Geometry: final body of the model. Coordinates: model frame, mm. A direction names the side the tool comes from. Round coordinates to 2 decimals unless told otherwise and drop trailing zeros. Write each loop counter-clockwise with the first axis right and the second up, starting at its lowest first coordinate (ties: lowest second). Pieces come first, ordered by that corner, then holes. Notation, with made-up numbers: (21.5, -34.75) -> (41.5, -34.75) arc R21 cw to (41.5, -19.75) -> close; hole circle Ø7 at (-11.75, 0). An arc over 180 degrees is marked (long way). Use one line per item in the form item = value. Start each with the question number.
1. Cut plane D-D, the plane y = -32. Return the cut outline in (x, z).
2. Reachability of faces 5 (the face through (5.734, -65.346, 70.392)), 6 (the face through (-5.116, -73.362, 8.112)), 7 (the face through (-8.075, -18, 2)), 8 (the face through (-6, -17, 16)) from +Z, -Z, +X, -X, +Y, -Y: full face, straight path, thin tool, end or side. Return the list, or none.
3. Draft query along Y for faces 1 (the face through (5.734, -62.007, 71.08)), 2 (the face through (-6, -77.2, 8)), 3 (the face through (-13, -46, 21)), 4 (the face through (-4, -23.65, 4)). Return one class per face: pulls with the +Y half, pulls with the -Y half, needs draft (parallel to the pull), parting line crosses it, or undercut.
4. Cut plane B-B, the plane x = -11. Return the cut outline in (y, z) (1 decimal).
5. Cut plane A-A, the plane x = -6.5. State how many separate pieces and enclosed holes the cut face has, plus the area to 3 significant figures.
6. Pin query (flat end, axial travel): pin 1 Ø10.5 at (x, y) = (-5.5, -65.5) entering from +Z; pin 2 Ø10 at (x, z) = (-3, 10.5) entering from -Y; pin 3 Ø8 at (x, y) = (-6.5, -70.7) entering from +Z. Return the tip coordinate at first contact, or that it passes through.
7. Line query: L1, parallel to Y at x = -6, z = 12; L2, parallel to Z at x = -8.5, y = -15.5; L3, parallel to X at y = -24.5, z = 3.5. Output: solid intervals per line, ascending.
```python
from build123d import *

# Parameters (mm, degrees)
F0_R      = 4.415
F0_W      = 3.025
F0_H      = 16
F0_W_2    = 7.0735459991
F1_DEPTH  = 13
F3_DEPTH  = 8.075
F4_R      = 10
F5_R      = 3
F6_DEPTH  = 25
F7_R      = 3.2
F8_DEPTH  = 11.1
F10_DEPTH = 25


# Not quite as in the source:
# - ends of sketch curves that miss each other by under 0.0002 mm in the source are joined


with BuildPart() as f1:
    # F0 (on Right) → F1 (new body)
    with BuildSketch(Plane.YZ):
        with BuildLine():
            Line((-11.2, 0), (0, 0))
            Line((0, 0), (0, 12))
            ThreePointArc((0, 12), (-1.1715728753, 14.8284271247), (-4, 16))
            Line((-4, 16), (-34.4146185314, 16))
            Line((-34.4146185314, 16), (-69.7679370642, 58.1324443715))
            Line((-69.7679370642, 58.1324443715), (-58.8383850945, 67.3034273983))
            Line((-58.8383850945, 67.3034273983), (-65.2662611913, 74.9638718294))
            Line((-65.2662611913, 74.9638718294), (-67.5643945207, 73.0355090004))
            Line((-67.5643945207, 73.0355090004), (-63.0648812529, 67.6731978986))
            Line((-63.0648812529, 67.6731978986), (-79.9178590015, 53.5318704855))
            Line((-79.9178590015, 53.5318704855), (-53.9387302293, 22.5711504387))
            ThreePointArc((-53.9387302293, 22.5711504387), (-53.3776768537, 18.309526953), (-57.0029080018, 16))
            Line((-57.0029080018, 16), (-67.1014540009, 16))
            Line((-67.1014540009, 16), (-67.1014540009, 0))
            Line((-67.1014540009, 0), (-64.0764540009, 0))
            Line((-64.0764540009, 0), (-23.65, 0))
            Line((-23.65, 0), (-23.65, 7.375))
            ThreePointArc((-23.65, 7.375), (-21.8267397129, 11.7767397129), (-17.425, 13.6))
            ThreePointArc((-17.425, 13.6), (-13.0232602871, 11.7767397129), (-11.2, 7.375))
            Line((-11.2, 7.375), (-11.2, 0))
        make_face()
        with BuildLine():
            Line((-23.65, 0), (-11.2, 0))
            Line((-11.2, 0), (-11.2, 7.375))
            ThreePointArc((-11.2, 7.375), (-13.0232602871, 11.7767397129), (-17.425, 13.6))
            ThreePointArc((-17.425, 13.6), (-21.8267397129, 11.7767397129), (-23.65, 7.375))
            Line((-23.65, 7.375), (-23.65, 0))
        make_face()
        with Locations((-17.425, 7.375)):
            Circle(F0_R, mode=Mode.SUBTRACT)
        with Locations((-68.6139540009, 8)):
            Rectangle(F0_W, F0_H)
        with Locations((-73.6632270005, 8)):
            Rectangle(F0_W_2, F0_H)
    extrude(amount=-F1_DEPTH)

    # F2 (on face) → F3 (cut)
    with BuildSketch(Plane.YZ):
        with BuildLine():
            Line((-17.425, 0), (-11.2, 0))
            Line((-11.2, 0), (-11.2, 7.3750006942))
            ThreePointArc((-11.2, 7.3750006942), (-11.2387169647, 8.068201392), (-11.3543862514, 8.7527792377))
            ThreePointArc((-11.3543862514, 8.7527792377), (-18.1182010341, 13.5612829976), (-23.65, 7.375))
            Line((-23.65, 7.375), (-23.65, 0))
            Line((-23.65, 0), (-17.425, 0))
        make_face()
        with BuildLine():
            ThreePointArc((-13.01, 7.375), (-14.3031235611, 4.2531235611), (-17.425, 2.96))
            ThreePointArc((-17.425, 2.96), (-20.5468764389, 10.4968764389), (-13.01, 7.375))
        make_face(mode=Mode.SUBTRACT)
    extrude(amount=-F3_DEPTH, mode=Mode.SUBTRACT)

    # F4
    f4_edges = [f1.edges().sort_by_distance(p)[0] for p in [
        (-6.5, -34.414619, 16),
    ]]
    fillet(f4_edges, radius=F4_R)

    # F5 (on face) → F6 (cut)
    with BuildSketch(Plane.XY.offset(16)):
        with Locations((-6.5, -70.7)):
            Circle(F5_R)
    extrude(amount=-F6_DEPTH, mode=Mode.SUBTRACT)

    # F7 (on face) → F8 (cut)
    with BuildSketch(Plane(origin=(0, -59.3794347551, 70.7656546956), x_dir=(1, 0, 0), z_dir=(0, -0.6427876097, 0.7660444431))):
        with Locations((-6.5, -10.8610087227)):
            Circle(F7_R)
    extrude(amount=-F8_DEPTH, mode=Mode.SUBTRACT)

    # F9 (on face) → F10 (join)
    with BuildSketch(Plane.YZ):
        Polygon((-77.9894961724, 51.2337371561), (-58.8383850945, 67.3034273983), (-65.2662611913, 74.9638718294), (-67.5643945207, 73.0355090004), (-63.0648812529, 67.6731978986), (-79.9178590015, 53.5318704855), align=None)
    extrude(amount=F10_DEPTH)


solid = f1.part
```
Outcome:
q1.outline = (-13, 0) -> (0, 0) -> (0, 16.26) -> (-13, 16.26) -> close
q2.face_5 = +X, -X, -Y
q2.face_6 = -Z
q2.face_7 = -Z, +X
q2.face_8 = +Z, +X, -X, +Y
q3.face_1 = pulls with the +Y half
q3.face_2 = pulls with the -Y half
q3.face_3 = needs draft
q3.face_4 = undercut
q4.outline = (-79.9, 53.5) -> (-53.9, 22.6) arc R4 cw to (-57, 16) -> (-77.2, 16) -> (-77.2, 0) -> (0, 0) -> (0, 12) arc R4 ccw to (-4, 16) -> (-29.8, 16) arc R10 cw to (-37.4, 19.6) -> (-69.8, 58.1) -> (-58.8, 67.3) -> (-65.3, 75) -> (-67.6, 73) -> (-63.1, 67.7) -> close; hole circle Ø8.8 at (-17.4, 7.4)
q5.separate_pieces = 3
q5.enclosed_holes = 0
q5.area = 1,620 mm^2
q6.pin_1 = 74.96
q6.pin_2 = -77.2
q6.pin_3 = 73.76
q7.L1 = -77.2 to -73.66, -67.74 to -21.59, -13.26 to 0
q7.L2 = 0 to 3.4, 11.35 to 16
q7.L3 = -13 to 0
